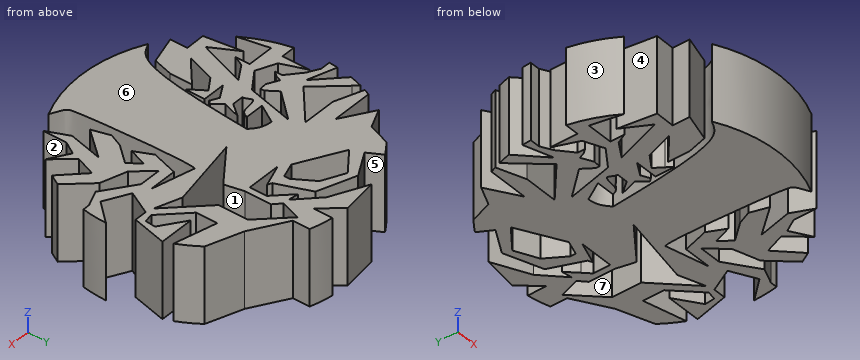
```python
from build123d import *

# Parameters (mm, degrees)
F1_DEPTH = 25.4


with BuildPart() as f1:
    # F0 (on Top) → F1 (new body)
    with BuildSketch(Plane.XY):
        with BuildLine():
            ThreePointArc((43.704676099, -8.1057872589), (44.2632768364, -4.0699906266), (44.45, 0))
            Line((44.45, 0), (38.3762454863, -6.7695145848))
            Line((38.3762454863, -6.7695145848), (30.4140662095, -2.5716401001))
            Line((30.4140662095, -2.5716401001), (34.4598693357, 5.1021028682))
            Line((34.4598693357, 5.1021028682), (38.5398091507, 5.1021028682))
            Line((38.5398091507, 5.1021028682), (41.340966117, 16.3317794656))
            Line((41.340966117, 16.3317794656), (29.7620025051, 16.3317794656))
            Line((29.7620025051, 16.3317794656), (37.6569107253, 10.7998840139))
            Line((37.6569107253, 10.7998840139), (37.3528477732, 7.4648817648))
            Line((37.3528477732, 7.4648817648), (34.4598693357, 7.0039533134))
            Line((34.4598693357, 7.0039533134), (26.3554092655, 15.3433524242))
            Line((26.3554092655, 15.3433524242), (26.3554092655, 22.3718555596))
            Line((26.3554092655, 22.3718555596), (40.1509507291, 19.0710161121))
            ThreePointArc((40.1509507291, 19.0710161121), (38.2404494141, 22.6598880979), (36.0100197183, 26.0591822567))
            Line((36.0100197183, 26.0591822567), (24.5059830732, 30.046253556))
            Line((24.5059830732, 30.046253556), (13.1523255345, 36.8548135049))
            Line((13.1523255345, 36.8548135049), (13.1523255345, 42.4596141414))
            ThreePointArc((13.1523255345, 42.4596141414), (9.520993243, 43.418350817), (5.8216881898, 44.0671129826))
            Line((5.8216881898, 44.0671129826), (5.8216881898, 37.7795321464))
            Line((5.8216881898, 37.7795321464), (0, 44.45))
            Line((0, 44.45), (-11.5668197775, 42.9186577171))
            Line((-11.5668197775, 42.9186577171), (0, 37.3720790271))
            Line((0, 37.3720790271), (7.0577384585, 30.3874456776))
            Line((7.0577384585, 30.3874456776), (3.6453471464, 30.9077701819))
            Line((3.6453471464, 30.9077701819), (7.0577384585, 27.3500500395))
            Line((7.0577384585, 27.3500500395), (9.3304236081, 25.0318586734))
            Line((9.3304236081, 25.0318586734), (9.3304236081, 19.3706885501))
            Line((9.3304236081, 19.3706885501), (-2.1026324375, 19.3706885501))
            Line((-2.1026324375, 19.3706885501), (5.5705367236, 22.0912819416))
            Line((5.5705367236, 22.0912819416), (4.2201406021, 22.7765895828))
            Line((4.2201406021, 22.7765895828), (0, 33.6315410045))
            Line((0, 33.6315410045), (-12.2639499105, 37.9127315635))
            Line((-12.2639499105, 37.9127315635), (-20.8245608606, 33.0582727561))
            Line((-20.8245608606, 33.0582727561), (-23.4805989564, 37.7420716528))
            ThreePointArc((-23.4805989564, 37.7420716528), (-25.7137068729, 36.2575203076), (-27.853233261, 34.6410146634))
            Line((-27.853233261, 34.6410146634), (-30.3483057479, 27.6229865325))
            Line((-30.3483057479, 27.6229865325), (-37.0270949757, 24.5926155108))
            Line((-37.0270949757, 24.5926155108), (-26.9607932241, 18.317772023))
            Line((-26.9607932241, 18.317772023), (-40.5001447913, 18.317772023))
            ThreePointArc((-40.5001447913, 18.317772023), (-40.9156869326, 17.3697744036), (-41.3090426286, 16.4123580605))
            Line((-41.3090426286, 16.4123580605), (-32.2220331053, 13.1766568099))
            Line((-32.2220331053, 13.1766568099), (-20.9865597638, 13.1766568099))
            Line((-20.9865597638, 13.1766568099), (-32.3342754558, 3.2778158817))
            Line((-32.3342754558, 3.2778158817), (-40.5535289611, 12.7001060929))
            Line((-40.5535289611, 12.7001060929), (-42.0881711734, 14.2964452671))
            ThreePointArc((-42.0881711734, 14.2964452671), (-42.7156199987, 12.2954588416), (-43.247994613, 10.2671058217))
            Line((-43.247994613, 10.2671058217), (-34.9080591648, 2.0286042741))
            Line((-34.9080591648, 2.0286042741), (-44.1701690125, 4.9798262425))
            ThreePointArc((-44.1701690125, 4.9798262425), (-44.311503506, 3.5061598702), (-44.4036852603, 2.0286042741))
            Line((-44.4036852603, 2.0286042741), (-41.0906250328, 2.0286042741))
            Line((-41.0906250328, 2.0286042741), (-37.3294337081, 0))
            Line((-37.3294337081, 0), (-32.6545804034, -4.0618134039))
            Line((-32.6545804034, -4.0618134039), (-32.6545804034, -6.4967229435))
            Line((-32.6545804034, -6.4967229435), (-31.4006268427, -5.0094540041))
            Line((-31.4006268427, -5.0094540041), (-30.6248067702, -3.1227373514))
            Line((-30.6248067702, -3.1227373514), (-26.9258844929, -5.0023249455))
            Line((-26.9258844929, -5.0023249455), (-24.6496018838, -4.7759504527))
            Line((-24.6496018838, -4.7759504527), (-24.680626463, -3.5207036625))
            Line((-24.680626463, -3.5207036625), (-27.1262085414, 0))
            Line((-27.1262085414, 0), (-19.111280333, 8.9932536787))
            Line((-19.111280333, 8.9932536787), (-22.8618391946, -6.1794005338))
            Line((-22.8618391946, -6.1794005338), (-29.4998778801, -10.790373226))
            Line((-29.4998778801, -10.790373226), (-35.8092829268, -8.075045983))
            Line((-35.8092829268, -8.075045983), (-38.8495844895, 0))
            Line((-38.8495844895, 0), (-38.8495844895, -9.0487861421))
            Line((-38.8495844895, -9.0487861421), (-43.5192137952, -9.0487861421))
            ThreePointArc((-43.5192137952, -9.0487861421), (-41.2439066607, -16.5753631444), (-37.6780041311, -23.5832674729))
            Line((-37.6780041311, -23.5832674729), (-39.6750552833, -13.5251467775))
            Line((-39.6750552833, -13.5251467775), (-30.8937566892, -13.5251467775))
            Line((-30.8937566892, -13.5251467775), (-30.8937566892, -18.2168473015))
            Line((-30.8937566892, -18.2168473015), (-29.2824792269, -14.9614370338))
            Line((-29.2824792269, -14.9614370338), (-23.8202681725, -11.5252173406))
            Line((-23.8202681725, -11.5252173406), (-29.2824792269, -26.9571319202))
            Line((-29.2824792269, -26.9571319202), (-34.0718732776, -18.2168473015))
            Line((-34.0718732776, -18.2168473015), (-32.4182662921, -30.4114864914))
            Line((-32.4182662921, -30.4114864914), (-26.0305313037, -30.3295583668))
            Line((-26.0305313037, -30.3295583668), (-26.0305313037, -36.0307360464))
            Line((-26.0305313037, -36.0307360464), (-16.6308986723, -33.2953852711))
            Line((-16.6308986723, -33.2953852711), (-14.8497161906, -26.9571319202))
            Line((-14.8497161906, -26.9571319202), (-14.8497161906, -19.681075499))
            Line((-14.8497161906, -19.681075499), (-23.2630656429, -26.9571319202))
            Line((-23.2630656429, -26.9571319202), (-20.0048710871, -17.7520353818))
            Line((-20.0048710871, -17.7520353818), (-15.5527187897, -14.7480303308))
            Line((-15.5527187897, -14.7480303308), (-13.5784722435, -17.6740062021))
            Line((-13.5784722435, -17.6740062021), (-12.1584481763, -19.5038274832))
            Line((-12.1584481763, -19.5038274832), (-12.1584481763, -13.2389037838))
            Line((-12.1584481763, -13.2389037838), (-19.6191504902, -13.2389037838))
            Line((-19.6191504902, -13.2389037838), (-15.0464561653, -10.5254098808))
            Line((-15.0464561653, -10.5254098808), (-12.3378359363, -11.8821568323))
            Line((-12.3378359363, -11.8821568323), (-11.3327408226, -10.7720452013))
            Line((-11.3327408226, -10.7720452013), (-13.8265134831, -7.7241360835))
            Line((-13.8265134831, -7.7241360835), (-12.014329364, -2.1424514692))
            Line((-12.014329364, -2.1424514692), (-15.1898814267, -6.1794005338))
            Line((-15.1898814267, -6.1794005338), (-18.8946343708, -6.1794005338))
            add(Edge.make_bspline(
                [(-13.2013149351, 0), (-13.5679742386, -0.867562918), (-14.1417802712, -2.8551336689), (-21.6731611335, -2.4070426946), (-18.8164656554, -4.9714057174), (-18.8946343708, -6.1794005338)],
                knots=[0, 0, 0, 0, 0.2937199062, 0.6908083029, 1, 1, 1, 1], degree=3))
            Line((-13.2013149351, 0), (-19.394499122, 0))
            Line((-19.394499122, 0), (-15.643126382, 6.2778336934))
            add(Edge.make_bspline(
                [(-9.2623769855, 3.1903743622), (-10.1683737145, 4.0650652939), (-11.9716685733, 5.8060491295), (-14.4232490293, 6.1210787108), (-15.643126382, 6.2778336934)],
                knots=[0, 0, 0, 0, 0.5024118627, 1, 1, 1, 1], degree=3))
            add(Edge.make_bspline(
                [(-20.8984651632, -39.2308125563), (-19.0227174729, -38.4354283736), (-12.6089325614, -35.6754345167), (-10.6492832076, -12.9029994524), (-9.2623769855, 3.1903743622)],
                knots=[0, 0, 0, 0, 0.2933422321, 1, 1, 1, 1], degree=3))
            ThreePointArc((-20.8984651632, -39.2308125563), (-1.4267302198, -44.4270969216), (18.3382861829, -40.4908602017))
            add(Edge.make_bspline(
                [(18.3382861829, -40.4908602017), (16.800650041, -39.7684573781), (13.8810869179, -38.3785879352), (12.7340809413, -36.0534150056), (10.8537079929, 4.3088263933), (12.4095863322, 3.2863546111), (12.5556673868, 3.1903743622)],
                knots=[0, 0, 0, 0, 0.1945745472, 0.3689525646, 0.9407210575, 1, 1, 1, 1], degree=3))
            Line((12.5556673868, 3.1903743622), (26.0327312476, 0))
            Line((26.0327312476, 0), (16.6674540937, 0))
            Line((16.6674540937, 0), (14.1163282306, -8.2934123817))
            Line((14.1163282306, -8.2934123817), (16.7920096617, -13.9933407127))
            Line((16.7920096617, -13.9933407127), (18.8650966271, -8.1886949246))
            Line((18.8650966271, -8.1886949246), (21.7674178411, -12.1275609654))
            Line((21.7674178411, -12.1275609654), (16.7920096617, -17.9322074255))
            Line((16.7920096617, -17.9322074255), (14.9226369154, -22.1807765402))
            Line((14.9226369154, -22.1807765402), (16.5846997555, -28.0903350345))
            Line((16.5846997555, -28.0903350345), (24.2551246189, -18.9687502362))
            Line((24.2551246189, -18.9687502362), (21.5601079349, -29.9561134378))
            Line((21.5601079349, -29.9561134378), (24.6297491832, -37.0024047215))
            Line((24.6297491832, -37.0024047215), (24.6297491832, -29.3928310512))
            Line((24.6297491832, -29.3928310512), (27.1574471769, -25.1880124765))
            Line((27.1574471769, -25.1880124765), (33.6225707529, -29.074477398))
            Line((33.6225707529, -29.074477398), (27.9866814255, -22.4929984806))
            Line((27.9866814255, -22.4929984806), (30.4743868592, -16.0664276781))
            Line((30.4743868592, -16.0664276781), (37.7759431419, -23.4260670993))
            ThreePointArc((37.7759431419, -23.4260670993), (38.783221777, -21.7178315814), (39.7133054721, -19.9663684349))
            Line((39.7133054721, -19.9663684349), (32.5474751687, -11.9202537473))
            Line((32.5474751687, -11.9202537473), (24.099831034, -9.3132333563))
            Line((24.099831034, -9.3132333563), (18.7873544042, -3.2667341875))
            Line((18.7873544042, -3.2667341875), (26.0327312476, -3.2667341875))
            Line((26.0327312476, -3.2667341875), (35.9974019018, -10.3736902339))
            Line((35.9974019018, -10.3736902339), (41.4131227431, -8.1057872589))
            Line((41.4131227431, -8.1057872589), (43.704676099, -8.1057872589))
        make_face()
        Polygon((-4.9189029301, 21.5841254968), (-19.2240415026, 29.2505866358), (-11.4039010319, 35.1327965548), (-4.1301422855, 31.6558589691), (0, 25.0814852009), (0, 23.2533977972), align=None, mode=Mode.SUBTRACT)
        Polygon((12.6878964172, 13.258886178), (11.3784278194, 19.3706885501), (11.3784278194, 28.1440664159), (9.0285656372, 30.3874456776), (11.3085236792, 36.8548135049), (20.1618225394, 27.6124433138), (20.1618225394, 17.8627432901), (31.941140432, 5.741956426), (23.5674446572, 8.5952473997), (0, 3.9316086214), align=None, mode=Mode.SUBTRACT)
    extrude(amount=F1_DEPTH)


solid = f1.part
```
Input: part model. Units: mm. Frame: model coordinates. Face numbers are marked on the shaded views. A direction names the side the tool comes from. Give positions to 0.01 mm unless a question says otherwise; leave off trailing zeros.
1. Draft query along Y for the marked faces 5, 6 and 7. Return one class per face: released by +Y, released by -Y, zero draft, split by the parting line, or undercut.
Computed:
face 5: released by +Y
face 6: zero draft
face 7: undercut
2. Pin query (flat end, axial travel): pin 1 Ø8 at (y, z) = (27.5, 20) entering from -X; pin 2 Ø3 at (y, z) = (-18, 16) entering from -X; pin 3 Ø7.5 at (x, z) = (21.5, 11) entering from +Y; pin 4 Ø1 at (x, y) = (22.5, -33) entering from -Z. Return the tip coordinate at first contact, or that it passes through.
Computed:
pin 1: stops at x = -37.03
pin 2: stops at x = -41.27
pin 3: stops at y = 34.1
pin 4: stops at z = 0
3. Line query: probe 1 along Y at (x, z) = (-8.5, 10); probe 2 along Y at (x, z) = (37, 16.75); probe 3 along Y at (x, z) = (27, 4.75). Output: solid intervals per line, ascending.
Computed:
probe 1: y = -43.63 to 23.5, 33.74 to 36.6, 41.45 to 43.32
probe 2: y = -22.64 to -16.92, -9.95 to -6.04, 5.1 to 7.41, 11.26 to 16.33, 19.82 to 24.63
probe 3: y = -25.45 to -10.21, -3.96 to 7.43, 10.83 to 14.68, 22.22 to 29.18
4. Set-up query: the marked faces 1, 2, 3 and 4. Return all of +Z, -Z, +X, -X, +Y, -Y with unobstructed straight access to the full face (end or side cutting, diameter ignored); none if empty.
Computed:
face 1: +Z, -Z
face 2: +Z, -Z, +X, -Y
face 3: +Z, -Z, -X, -Y
face 4: +Z, -Z, -Y
5. Cut plane A-A (z = 4). State how many separate pieces and enclosed holes the cut face has, and give its area (3 significant figures).
Computed:
separate pieces: 1
enclosed holes: 2
area: 3,850 mm2
